Build history of the part. All positions in model axes, mm. Face numbers are marked on the shaded views. A direction names the side the tool comes from. Round coordinates to 2 decimals unless told otherwise and drop trailing zeros. Write each loop counter-clockwise with the first axis right and the second up, starting at its lowest first coordinate (ties: lowest second). Pieces come first, ordered by that corner, then holes. Notation, with made-up numbers: (-35.5, 72) -> (-29.5, 72) arc R25 ccw to (-29.5, 94) -> close; hole circle Ø3 at (37.5, 88.5). An arc over 180 degrees is marked (long way). One line per question, with ' | ' between items.
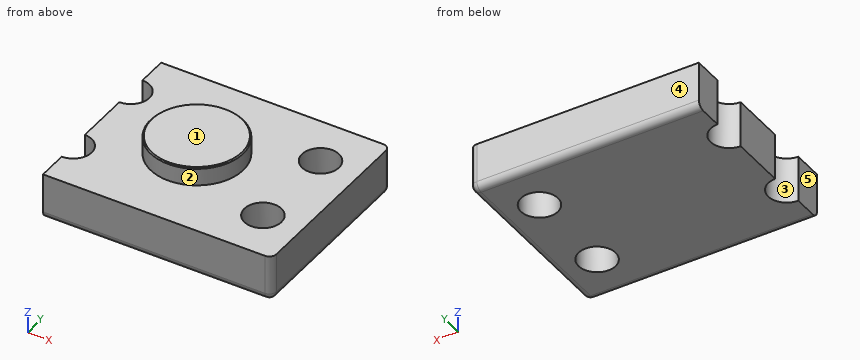
from build123d import *

# Parameters (mm, degrees)
BOSS_EXTRUDE1_DEPTH = 20
SKETCH2_R           = 8
CUT_EXTRUDE1_DEPTH  = 21
LPATTERN1_COUNT     = 2
LPATTERN1_PITCH     = 40
SKETCH3_R           = 20
BOSS_EXTRUDE2_DEPTH = 8
CHAMFER1_SIZE       = 0.5
FILLET1_R           = 3


with BuildPart() as part:
    # Sketch1 → Boss-Extrude1 (new body)
    with BuildSketch(Plane.XY):
        with BuildLine():
            Line((0, 69), (0, 82))
            Line((0, 82), (99, 82))
            Line((99, 82), (99, 0))
            Line((99, 0), (0, 0))
            Line((0, 0), (0, 13))
            ThreePointArc((0, 13), (8, 21), (0, 29))
            Line((0, 29), (0, 53))
            ThreePointArc((0, 53), (8, 61), (0, 69))
        make_face()
    extrude(amount=BOSS_EXTRUDE1_DEPTH)

    # Sketch2 → Cut-Extrude1 (cut, through all)
    with BuildSketch(Plane.XY.offset(20)):
        with Locations((82, 21)):
            Circle(SKETCH2_R)
    cut_extrude1 = extrude(amount=-CUT_EXTRUDE1_DEPTH, mode=Mode.SUBTRACT)

    # LPattern1: Cut-Extrude1 ×2
    with Locations(*[(0, i * LPATTERN1_PITCH, 0) for i in range(1, LPATTERN1_COUNT)]):
        add(cut_extrude1, mode=Mode.SUBTRACT)

    # Sketch3 → Boss-Extrude2 (add)
    with BuildSketch(Plane.XY.offset(20)):
        with Locations((41, 41)):
            Circle(SKETCH3_R)
    extrude(amount=BOSS_EXTRUDE2_DEPTH)

    # Chamfer1
    chamfer1_edges = [part.edges().sort_by_distance(p)[0] for p in [
        (21, 41, 28),
    ]]
    chamfer(chamfer1_edges, length=CHAMFER1_SIZE)

    # Fillet1
    fillet1_edges = [part.edges().sort_by_distance(p)[0] for p in [
        (49.5, 82, 0),
        (99, 41, 0),
        (49.5, 0, 0),
        (99, 82, 10),
        (99, 0, 10),
    ]]
    fillet(fillet1_edges, radius=FILLET1_R)


solid = part.part
(1) 3-axis set-ups, long thin cutter, end or side, ignore diameter. For the marked faces 1 and 2: which of +Z, -Z, +X, -X, +Y, -Y reach the whole face in a straight line?
Calculated:
face 1: +Z, +X, -X, +Y, -Y | face 2: +Z
(2) Drop flat-ended pins along their axis: pin 1 (8 mm diameter, centred on x = 78, y = 29.5, fed in from -Z); pin 2 (18.5 mm diameter, centred on x = 82, y = 21, fed in from +Z); pin 3 (9.5 mm diameter, centred on x = 82, y = 61, fed in from +Z). Give the stop position or say it passes through.
Calculated:
pin 1: z = 0 | pin 2: z = 20 | pin 3: through
(3) Slice it at B-B (z = 4.25). Write the cut outline in (x, y), then the cut area to 3 significant figures.
Calculated:
outline: (0, 0) -> (96, 0) arc R3 ccw to (99, 3) -> (99, 79) arc R3 ccw to (96, 82) -> (0, 82) -> (0, 69) arc R8 cw to (0, 53) -> (0, 29) arc R8 cw to (0, 13) -> close; hole circle Ø16 at (82, 21); hole circle Ø16 at (82, 61) | area: 7,510 mm2
(4) Slice it at A-A (x = 82). Write the cut outline in (y, z), then the cut area to 3 significant figures.
Calculated:
outline: (0, 3) arc R3 ccw to (3, 0) -> (13, 0) -> (13, 20) -> (0, 20) -> close; (29, 0) -> (53, 0) -> (53, 20) -> (29, 20) -> close; (69, 0) -> (79, 0) arc R3 ccw to (82, 3) -> (82, 20) -> (69, 20) -> close | area: 996 mm2
(5) Mould opens along Y. For the marked faces 3, 4 and 5 say: pulls with the +Y half, pulls with the -Y half, needs draft (parallel to the pull), parting line crosses it, or undercut.
Calculated:
face 3: undercut | face 4: pulls with the +Y half | face 5: needs draft
(6) Wall check: line 1 (Y direction, x = 82, z = 11); line 2 (Y direction, x = 76.5, z = 14.5); line 3 (Z direction, x = 88.5, y = 78.5). Give the ranges that are in metal, low to high. Write a range as from..to.
Calculated:
line 1: 0..13, 29..53, 69..82 | line 2: 0..15.19, 26.81..55.19, 66.81..82 | line 3: 0..20
(7) Slice it at C-C (y = 63.5). Write the cut outline in (x, z).
Calculated:
outline: (7.6, 0) -> (74.4, 0) -> (74.4, 20) -> (7.6, 20) -> close; (89.6, 0) -> (96, 0) arc R3 ccw to (99, 3) -> (99, 20) -> (89.6, 20) -> close
(8) Slice it at D-D (y = 41). Write the cut outline in (x, z), then the cut area to 3 significant figures.
Calculated:
outline: (0, 0) -> (96, 0) arc R3 ccw to (99, 3) -> (99, 20) -> (61, 20) -> (61, 27.5) -> (60.5, 28) -> (21.5, 28) -> (21, 27.5) -> (21, 20) -> (0, 20) -> close | area: 2,300 mm2
